Check sheet for the modelled part. Datum: model origin and axes. Units: mm. Round coordinates to 2 decimals unless told otherwise and drop trailing zeros. Order: outer loops, then holes, each group sorted by start corner. A loop starts at its lowest first (then second) coordinate and runs counter-clockwise, first axis right, second up.
Q1. Cross-section at B-B on x = -86. Record the cut outline in (y, z), then the cut area to 3 significant figures.
Q2. Scan lines: probe 1 along Z at (x, y) = (-55, -35); probe 2 along X at (y, z) = (-50, 80.5); probe 3 along Z at (x, y) = (-105, -44.5). Record each from-to range of solid material in increasing order.
Q3. Cross-section at C-C on z = -26.5. Record the cut outline in (x, y).
Q4. Depth check by flat-ended pin: P1, Ø2, axis at x = -2, z = 41, coming from the +Y side; P2, Ø2, axis at x = 24.5, y = -32, coming from the -Z side; P3, Ø8, axis at y = -63, z = 3.5, coming from the +X side; P4, Ø1, axis at x = -55.5, y = -32.5, coming from the +Z side. Enter the tip coordinate at first touch or a pass-through.
Q5. Cross-section at A-A on y = -29.5. Record the cut outline in (x, z).
from build123d import *

# Parameters (mm, degrees)
F1_DEPTH = 101.6


with BuildPart() as f1:
    # F0 (on Front) → F1 (new body)
    with BuildSketch(Plane.XZ):
        with BuildLine():
            Line((68.37305, 132.235599), (-16.435547, 132.235599))
            ThreePointArc((-16.435547, 132.235599), (-88.277596, 102.477647), (-118.035547, 30.635599))
            Line((-118.035547, 30.635599), (-118.035547, -39.357398))
            Line((-118.035547, -39.357398), (17.57305, -39.357398))
            ThreePointArc((17.57305, -39.357398), (53.494074, -24.478422), (68.37305, 11.442602))
            Line((68.37305, 11.442602), (68.37305, 132.235599))
        make_face()
    extrude(amount=F1_DEPTH)


solid = f1.part
Results found:
1. outline: (-101.6, -39.36) - (0, -39.36) - (0, 104.69) - (-101.6, 104.69) - close
1. area: 14,600 mm2
2. probe 1: z = -39.36 to 124.63
2. probe 2: x = -104.96 to 68.37
2. probe 3: z = -39.36 to 80.42
3. outline: (-118.04, -101.6) - (51.35, -101.6) - (51.35, 0) - (-118.04, 0) - close
4. P1: stops at y = 0
4. P2: stops at z = -39.01
4. P3: stops at x = 68.22
4. P4: stops at z = 124.63
5. outline: (-118.04, -39.36) - (17.57, -39.36) arc R50.8 ccw to (68.37, 11.44) - (68.37, 132.24) - (-16.44, 132.24) arc R101.6 ccw to (-118.04, 30.64) - close
